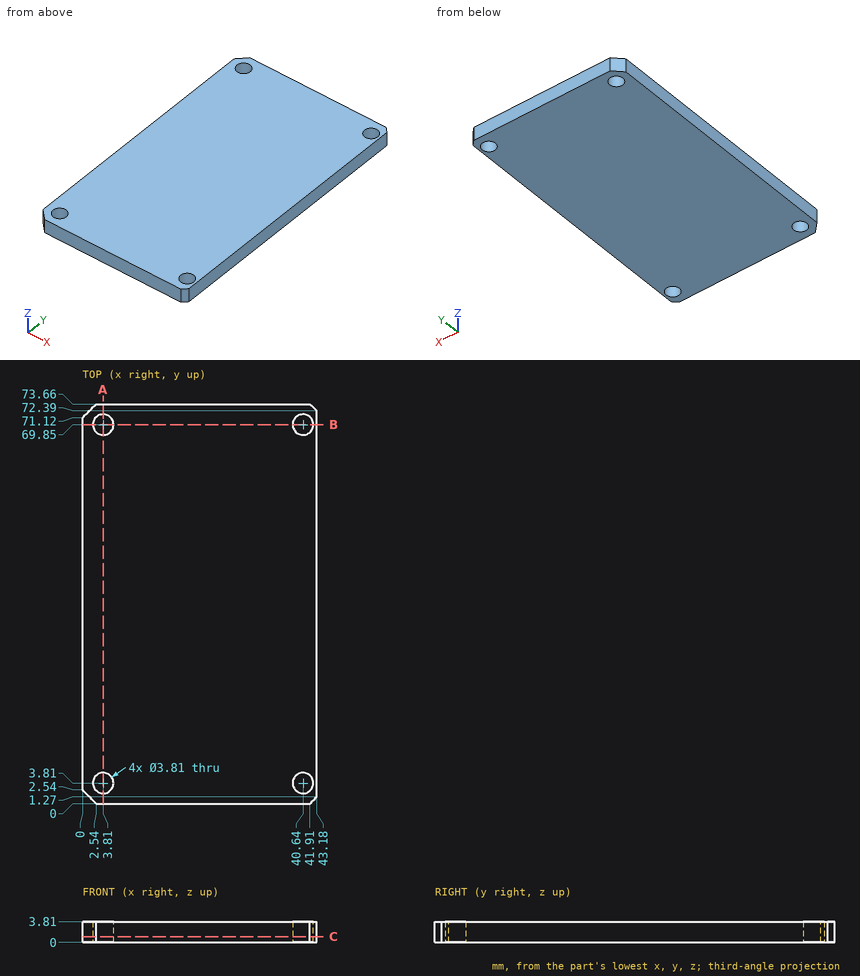
Study the drawing (mm; zero at the part's minimum x, y, z) and answer. Coordinates: 2 decimals unless noted, no trailing zeros. Loops run counter-clockwise (first coordinate to the right, second up) from the corner with the lowest first, then second, coordinate; pieces in that order, holes last. Notation, with made-up numbers: M -26,57.5 L -14,57.5 A25 cw -14,83.5 Z; hole C 34,67.25 d4. An arc over 180 degrees is marked long. Answer in a Markdown table with one row per item. Add a question column.
1. Find section C-C, the plane z = 1.05. Write down the section's boundary in (x, y) (3 decimals).
2. Find section A-A, the plane x = 3.81. Write down the section's boundary in (y, z) (3 decimals).
3. Find section B-B, the plane y = 69.85. Write down the section's boundary in (x, z) (3 decimals), then the cut area to 3 significant figures.
4. Consider L1, parallel to Y at x = 3.81, z = 1.35 (3 decimals); L2, parallel to X at y = 69.85, z = 1.6 (3 decimals). Determine where each line is inside the solid, lowest interval first.
Reported:
| question | item | result |
|---|---|---|
| 1 | outline | M 0,2.54 L 2.54,0 L 41.91,0 L 43.18,1.27 L 43.18,72.39 L 41.91,73.66 L 2.54,73.66 L 0,71.12 Z; hole C 3.81,3.81 d3.81; hole C 3.81,69.85 d3.81; hole C 40.64,3.81 d3.81; hole C 40.64,69.85 d3.81 |
| 2 | outline | M 0,0 L 1.905,0 L 1.905,3.81 L 0,3.81 Z; M 5.715,0 L 67.945,0 L 67.945,3.81 L 5.715,3.81 Z; M 71.755,0 L 73.66,0 L 73.66,3.81 L 71.755,3.81 Z |
| 3 | outline | M 0,0 L 1.905,0 L 1.905,3.81 L 0,3.81 Z; M 5.715,0 L 38.735,0 L 38.735,3.81 L 5.715,3.81 Z; M 42.545,0 L 43.18,0 L 43.18,3.81 L 42.545,3.81 Z |
| 3 | area | 135 mm^2 |
| 4 | L1 | y = 0 to 1.905, 5.715 to 67.945, 71.755 to 73.66 |
| 4 | L2 | x = 0 to 1.905, 5.715 to 38.735, 42.545 to 43.18 |
